The listing builds one solid part. Answer for the finished solid, in the listing's coordinates (mm). Face numbers are marked on the shaded views. A direction names the side the tool comes from. Coordinates: 2 decimals unless noted, no trailing zeros. Order: outer loops, then holes, each group sorted by start corner. A loop starts at its lowest first (then second) coordinate and runs counter-clockwise, first axis right, second up. Notation, with made-up numbers: (-9.75, 37) -> (-5.75, 37) arc R26 cw to (-5.75, 54) -> close; hole circle Ø6 at (54.5, -7). An arc over 180 degrees is marked (long way). Return JSON: item names as keys, results as strings.
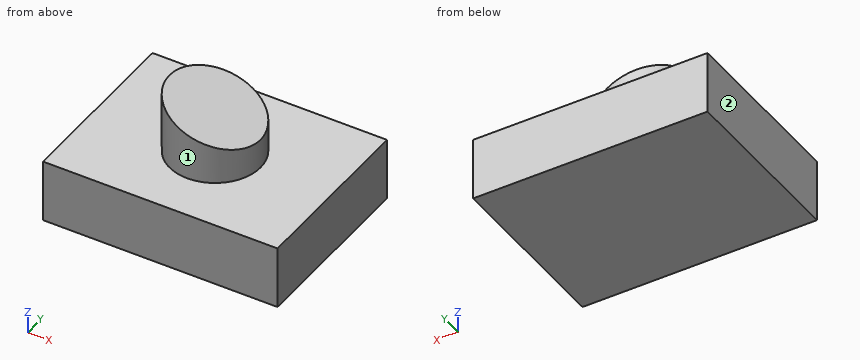
```python
from build123d import *

# Parameters (mm, degrees)
F0_W          = 94.798579812
F0_H          = 72.4261179566
F1_DEPTH      = 25.4
F2_R          = 18.3997173806
F3_DEPTH      = 25.4
F5_DEPTH      = 36.2140589783
F5_DEPTH_BACK = 36.2140589783


with BuildPart() as f1:
    # F0 (on Top) → F1 (new body)
    with BuildSketch(Plane.XY):
        Rectangle(F0_W, F0_H)
    extrude(amount=F1_DEPTH)

    # F2 (on face) → F3 (join)
    with BuildSketch(Plane.XY.offset(25.4)):
        Circle(F2_R)
    extrude(amount=F3_DEPTH)

    # F4 (on Front) → F5 (cut, two sides)
    with BuildSketch(Plane.XZ) as f5_sk:
        Polygon((19.6720566601, 52.7677323434), (-19.1493127495, 51.1912330985), (19.6720566601, 37.0027127904), align=None)
    extrude(amount=-F5_DEPTH, mode=Mode.SUBTRACT)
    extrude(f5_sk.sketch, amount=F5_DEPTH_BACK, mode=Mode.SUBTRACT)


solid = f1.part
```
Item 1: The part is cut by section B-B on x = 12. Determine the outline of the cut face in (y, z), plus the area to 3 significant figures.
Answer list:
{"outline": "(-36.21, 0) -> (36.21, 0) -> (36.21, 25.4) -> (13.95, 25.4) -> (13.95, 39.81) -> (-13.95, 39.81) -> (-13.95, 25.4) -> (-36.21, 25.4) -> close", "area": "2,240 mm2"}
Item 2: Flat-ended cylindrical pins translate along their axes: pin 1 (12 mm diameter, centred on x = 0.5, y = -14.5, fed in from +Z); pin 2 (6 mm diameter, centred on y = 1.5, z = 38.5, fed in from -X); pin 3 (6 mm diameter, centred on x = -5, z = 36.5, fed in from +Y); pin 4 (8 mm diameter, centred on y = -16.5, z = 28.5, fed in from -X). Find the tip coordinate at first contact, or state that the pin passes through.
Answer list:
{"pin 1": "z = 46.2", "pin 2": "x = -18.4", "pin 3": "y = 18.29", "pin 4": "x = -47.4"}
Item 3: Which of the six approach directions +Z, -Z, +X, -X, +Y, -Y give full straight-line access (tool end or side, diameter ignored) to the marked faces 1 and 2?
Answer list:
{"face 1": "+Z", "face 2": "+Z, -Z, -X, +Y, -Y"}
Item 4: Find the intervals of material crossed by probe 1 along Z at (x, y) = (-19, 11.5); probe 2 along Y at (x, z) = (2.5, 25.5); probe 3 along X at (y, z) = (-16.5, 32.5), in increasing order.
Answer list:
{"probe 1": "0 to 25.4", "probe 2": "-18.23 to 18.23", "probe 3": "-8.14 to 8.14"}
Item 5: The part is cut by section C-C on z = 33.5. Determine the outline of the cut face in (x, y).
Answer list:
{"outline": "circle Ø36.8 at (0, 0)"}
Item 6: The part is cut by section D-D on x = -13.5. Determine the outline of the cut face in (y, z).
Answer list:
{"outline": "(-36.21, 0) -> (36.21, 0) -> (36.21, 25.4) -> (12.5, 25.4) -> (12.5, 49.13) -> (-12.5, 49.13) -> (-12.5, 25.4) -> (-36.21, 25.4) -> close"}
Item 7: The part is cut by section A-A on y = 0. Determine the outline of the cut face in (x, z).
Answer list:
{"outline": "(-47.4, 0) -> (47.4, 0) -> (47.4, 25.4) -> (18.4, 25.4) -> (18.4, 37.47) -> (-18.08, 50.8) -> (-18.4, 50.8) -> (-18.4, 25.4) -> (-47.4, 25.4) -> close"}
